Design review of the part built by this model. Coordinates are the model's own, in mm. Face numbers are marked on the shaded views. A direction names the side the tool comes from. Coordinates: 2 decimals unless noted, no trailing zeros. Write each loop counter-clockwise with the first axis right and the second up, starting at its lowest first coordinate (ties: lowest second). Pieces come first, ordered by that corner, then holes. Notation, with made-up numbers: (84.5, 2.5) - (107.5, 2.5) arc R30 ccw to (107.5, 32.5) - close; hole circle Ø7 at (-22, 20.5). An arc over 180 degrees is marked (long way). Answer as CSV lines item,"result". Start each with the question number.
Q1. Clearance check with flat-ended pins moving along their axes: pin 1 (12 mm diameter, centred on x = -42.5, z = 19.5, fed in from +Y); pin 2 (5 mm diameter, centred on x = -26, z = 21.5, fed in from -Y); pin 3 (1 mm diameter, centred on y = -4.5, z = 20.5, fed in from -X); pin 4 (12 mm diameter, centred on x = -16, z = 43.5, fed in from -Y). State where each tip first meets the part, or that it passes through.
Q2. Machinability: for the marked faces 1, 2 and 3, which of the approach directions +Z, -Z, +X, -X, +Y, -Y give a long, thin tool a straight path to every point of the face, cutting with its end or side? Answer none if there is none.
Q3. We need section A-A (y = 0). Write out the cut boundary in (x, z), plus the area to 3 significant figures.
Q4. We need section B-B (z = 40.5). Write out the cut boundary in (x, y).
Q5. We need section C-C (x = -57.5). Write out the cut boundary in (y, z).
Q6. For line 1 along Y through (x, z) = (70.5, 7.25); line 2 along Z through (x, y) = (-22.25, 0); line 3 along Y through (x, z) = (70, 7), list the stretches that pass through material, from the lowest coordinate up. Write a range as [from, to].
Q7. We need section D-D (y = -22.5). Write out the cut boundary in (x, z).
from build123d import *

# Parameters (mm, degrees)
SKETCH_2_W          = 150
SKETCH_2_H          = 100
EXTRUDE_1_DEPTH     = 10
SKETCH_3_W          = 10
SKETCH_3_H          = 40
EXTRUDE_2_DEPTH     = 35
SKETCH_4_R          = 20
EXTRUDE_3_DEPTH     = 10
SKETCH_5_R          = 9.5
CUT_EXTRUDE_1_DEPTH = 10
M3X0_5_2_D          = 2.5


with BuildPart() as part:
    # ｽｹｯﾁ2 → ﾎﾞｽ - 押し出し1 (new body)
    with BuildSketch(Plane.XY):
        Rectangle(SKETCH_2_W, SKETCH_2_H)
    extrude(amount=EXTRUDE_1_DEPTH)

    # ｽｹｯﾁ3 → ﾎﾞｽ - 押し出し2 (add)
    with BuildSketch(Plane.XY):
        with Locations((-25, 0)):
            Rectangle(SKETCH_3_W, SKETCH_3_H)
    extrude(amount=EXTRUDE_2_DEPTH)

    # ｽｹｯﾁ4 → ﾎﾞｽ - 押し出し3 (add)
    with BuildSketch(Plane.ZY.offset(30)):
        with Locations((35, 0)):
            Circle(SKETCH_4_R)
    extrude(amount=-EXTRUDE_3_DEPTH)

    # ｽｹｯﾁ5 → ｶｯﾄ - 押し出し1 (cut)
    with BuildSketch(Plane.ZY.offset(30)):
        with Locations(Location((35, 0, 0), (0, 0, 270))):
            Circle(SKETCH_5_R)
    extrude(amount=-CUT_EXTRUDE_1_DEPTH, mode=Mode.SUBTRACT)

    # M3x0.5 ねじ穴2 (through all)
    with Locations(Plane.XY.offset(10)):
        with Locations((70.5, -10.000898701), (70.5, 29.999101299)):
            Hole(M3X0_5_2_D / 2)


solid = part.part
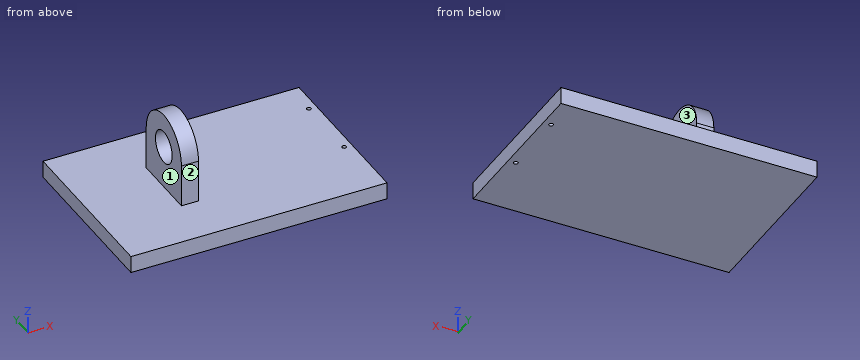
Results list:
1,pin 1,"passes through"
1,pin 2,"stops at y = -20"
1,pin 3,"stops at x = -30"
1,pin 4,"stops at y = -19.59"
2,face 1,"+Z, -X, +Y, -Y"
2,face 2,"+Z, +X, -X, -Y"
2,face 3,"+Z, +X, +Y, -Y"
3,outline,"(-75, 0) - (75, 0) - (75, 10) - (-20, 10) - (-20, 25.5) - (-30, 25.5) - (-30, 10) - (-75, 10) - close; (-30, 44.5) - (-20, 44.5) - (-20, 55) - (-30, 55) - close"
3,area,"1,760 mm2"
4,outline,"(-30, -19.23) - (-20, -19.23) - (-20, -7.75) - (-30, -7.75) - close; (-30, 7.75) - (-20, 7.75) - (-20, 19.23) - (-30, 19.23) - close"
5,outline,"(-50, 0) - (50, 0) - (50, 10) - (-50, 10) - close"
6,line 1,"y = [-50, -11.25], [-8.75, 28.75], [31.25, 50]"
6,line 2,"z = [0, 25.5], [44.5, 55]"
6,line 3,"y = [-50, -11.15], [-8.86, 28.85], [31.14, 50]"
7,outline,"(-75, 0) - (75, 0) - (75, 10) - (-75, 10) - close"
